Verification items for the finished model (mm, model axes). A direction names the side the tool comes from. Coordinates: 2 decimals unless noted, no trailing zeros. Write each loop counter-clockwise with the first axis right and the second up, starting at its lowest first coordinate (ties: lowest second). Pieces come first, ordered by that corner, then holes. Notation, with made-up numbers: (61, 63) -> (83, 63) arc R9 ccw to (83, 75) -> close; hole circle Ø9 at (21, -7.5). An arc over 180 degrees is marked (long way). Use a Markdown table: item, result. Add a question column.
from build123d import *

# Parameters (mm, degrees)
ESQUISSE1_R      = 2.5
EXTRUSION1_DEPTH = 3
CONG_1_R         = 10


with BuildPart() as part:
    # Esquisse1 → Extrusion1 (new body)
    with BuildSketch(Plane(origin=(0, 0, 0), x_dir=(1, 0, 0), z_dir=(0, 1, 0))):
        with BuildLine():
            Line((165, 0), (-165, 0))
            Line((-165, 0), (-165, -210))
            Line((-165, -210), (-147, -210))
            Line((-147, -210), (-132, -195))
            Line((-132, -195), (-132, -184))
            Line((-132, -184), (-100, -184))
            Line((-100, -184), (-63.363257782, -156.27367461))
            ThreePointArc((-63.363257782, -156.27367461), (0, -135), (63.363257782, -156.27367461))
            Line((63.363257782, -156.27367461), (100, -184))
            Line((100, -184), (132, -184))
            Line((132, -184), (132, -195))
            Line((132, -195), (147, -210))
            Line((147, -210), (165, -210))
            Line((165, -210), (165, 0))
        make_face()
        with Locations((-153, -12)):
            Circle(ESQUISSE1_R, mode=Mode.SUBTRACT)
        with Locations((153, -12)):
            Circle(ESQUISSE1_R, mode=Mode.SUBTRACT)
        with Locations((-153, -198)):
            Circle(ESQUISSE1_R, mode=Mode.SUBTRACT)
        with Locations((153, -198)):
            Circle(ESQUISSE1_R, mode=Mode.SUBTRACT)
        with Locations((-153, -111)):
            Circle(ESQUISSE1_R, mode=Mode.SUBTRACT)
        with Locations((153, -111)):
            Circle(ESQUISSE1_R, mode=Mode.SUBTRACT)
    extrude(amount=EXTRUSION1_DEPTH)

    # Congé1
    cong_1_edges = [part.edges().sort_by_distance(p)[0] for p in [
        (-165, 1.5, 0),
        (165, 1.5, 0),
        (165, 1.5, 210),
        (-165, 1.5, 210),
    ]]
    fillet(cong_1_edges, radius=CONG_1_R)


solid = part.part
1) Cross-section at D-D on x = -55. Record the boundary of the cut face in (y, z), then the cut area to 3 significant figures.
2) Release check for a two-part mould opening along X. For faces 1 (the face through (-161.99, 1.52, 2.85)), 2 (the face through (161.99, 1.52, 2.85)), 3 (the face through (-0.952, 1.479, 135.004)), 4 (the face through (81.425, 1.479, 169.943)) record: released by +X, released by -X, zero draft, split by the parting line, or undercut.
3) Cross-section at B-B on z = 141. Record the boundary of the cut face in (x, y), then the cut area to 3 significant figures.
4) Thickness scan on L1, parallel to Z at x = 153, y = 1.9; L2, parallel to X at y = 1.9, z = 12; L3, parallel to X at y = 1.1, z = 198. Record the ranges inside material, lowest first.
5) Cross-section at A-A on y = 1.8. Record the boundary of the cut face in (x, z), then the cut area to 3 significant figures.
6) Set-up check for faces 5 (the face through (-140, 1, 203)), 6 (the face through (-2, 0, 80)): record each of +Z, -Z, +X, -X, +Y, -Y from which the full face is reachable in a straight line by a thin tool's end or side.
7) Gauge pin test, flat ends, axial feed: pin 1 (6.5 mm diameter, centred on x = -153, z = 111, fed in from +Y); pin 2 (0.9 mm diameter, centred on x = -109.5, y = 2, fed in from +Z). Record the tip position at first contact, or that the pin passes through.
8) Cross-section at C-C on x = 74. Record the boundary of the cut face in (y, z), then the cut area to 3 significant figures.
Returned:
| question | item | result |
|---|---|---|
| 1 | outline | (0, 0) -> (3, 0) -> (3, 150.56) -> (0, 150.56) -> close |
| 1 | area | 452 mm² |
| 2 | face 1 | released by -X |
| 2 | face 2 | released by +X |
| 2 | face 3 | undercut |
| 2 | face 4 | undercut |
| 3 | outline | (-165, 0) -> (-34.99, 0) -> (-34.99, 3) -> (-165, 3) -> close; (34.99, 0) -> (165, 0) -> (165, 3) -> (34.99, 3) -> close |
| 3 | area | 780 mm² |
| 4 | L1 | z = 0 to 9.5, 14.5 to 108.5, 113.5 to 195.5, 200.5 to 210 |
| 4 | L2 | x = -165 to -155.5, -150.5 to 150.5, 155.5 to 165 |
| 4 | L3 | x = -165 to -155.5, -150.5 to -135, 135 to 150.5, 155.5 to 165 |
| 5 | outline | (-165, 10) arc R10 ccw to (-155, 0) -> (155, 0) arc R10 ccw to (165, 10) -> (165, 200) arc R10 ccw to (155, 210) -> (147, 210) -> (132, 195) -> (132, 184) -> (100, 184) -> (63.36, 156.27) arc R105 cw to (-63.36, 156.27) -> (-100, 184) -> (-132, 184) -> (-132, 195) -> (-147, 210) -> (-155, 210) arc R10 ccw to (-165, 200) -> close; hole circle Ø5 at (-153, 12); hole circle Ø5 at (-153, 111); hole circle Ø5 at (-153, 198); hole circle Ø5 at (153, 12); hole circle Ø5 at (153, 111); hole circle Ø5 at (153, 198) |
| 5 | area | 55,600 mm² |
| 6 | face 5 | +Z, +Y, -Y |
| 6 | face 6 | +Z, -Z, +X, -X, -Y |
| 7 | pin 1 | stops at y = 3 |
| 7 | pin 2 | stops at z = 184 |
| 8 | outline | (0, 0) -> (3, 0) -> (3, 164.32) -> (0, 164.32) -> close |
| 8 | area | 493 mm² |
